```python
from build123d import *

# Parameters (mm, degrees)
F2_R = 12.7
F4_R = 2.54


# Not quite as in the source:
# - a fillet or chamfer that OpenCascade refuses, or shapes differently, is made with other operations: its cross-section is extruded or revolved along the edge and cut away or added


with BuildPart() as f1:
    # F0 (on Front) → F1 (revolve)
    with BuildSketch(Plane.XZ):
        Polygon((53.5, 27), (-30.1052267423, 27), (-40.7862067223, 8.5), (-48.5, 8.5), (-48.5, 10), (-53.5, 10), (-53.5, 6.5), (-39.6315061839, 6.5), (-28.9505262039, 25), (51.5, 25), (51.5, 0), (53.5, 0), align=None)
    revolve(axis=Axis((0, 0, 0), (1, 0, 0)))

    # F2
    f2_edges = [f1.edges().sort_by_distance(p)[0] for p in [
        (-30.105227, 0, -27),
        (-28.950526, 0, -25),
    ]]
    fillet(f2_edges, radius=F2_R)

    # F3: fillet of radius 5.08 on 2 edges, made by hand

    # F3_s1 → F3_t2 (revolve)
    with BuildSketch(Plane.XZ):
        with BuildLine():
            ThreePointArc((-43.7191460897, 8.5), (-41.1791460897, 9.1805909488), (-39.3197370385, 11.04))
            Line((-39.3197370385, 11.04), (-40.7862067223, 8.5))
            Line((-40.7862067223, 8.5), (-43.7191460897, 8.5))
        make_face()
    revolve(axis=Axis((-40.7862067223, 0, 0), (1, 0, 0)))

    # F3_s3 → F3_t4 (revolve)
    with BuildSketch(Plane.XZ):
        with BuildLine():
            ThreePointArc((-48.5, 10), (-46.8477578714, 8.8899680172), (-44.8958357418, 8.5))
            Line((-44.8958357418, 8.5), (-48.5, 8.5))
            Line((-48.5, 8.5), (-48.5, 10))
        make_face()
    revolve(axis=Axis((-48.5, 0, 0), (1, 0, 0)))

    # F4
    f4_edges = [f1.edges().sort_by_distance(p)[0] for p in [
        (-48.5, 0, -10),
        (-53.5, 0, -10),
    ]]
    fillet(f4_edges, radius=F4_R)

    # F5: fillet of radius 2.54 on 1 edges, made by hand

    # F5_s1 → F5_t2 (revolve, cut)
    with BuildSketch(Plane.XZ):
        with BuildLine():
            ThreePointArc((-53.5, 7.46), (-52.6154054362, 6.7525560116), (-51.5112315369, 6.5))
            Line((-51.5112315369, 6.5), (-53.5, 6.5))
            Line((-53.5, 6.5), (-53.5, 7.46))
        make_face()
    revolve(axis=Axis((-53.5, 0, 0), (1, 0, 0)), mode=Mode.SUBTRACT)


solid = f1.part
```
Check sheet for the modelled part. Datum: model origin and axes. Units: mm. A direction names the side the tool comes from. Coordinates: 2 decimals unless noted, no trailing zeros. Order: outer loops, then holes, each group sorted by start corner. A loop starts at its lowest first (then second) coordinate and runs counter-clockwise, first axis right, second up. Notation, with made-up numbers: M -20.5,5 L 38.5,5 A13 cw 38.5,30 Z; hole C 72,-8.75 d1. An arc over 180 degrees is marked long. Write each question's results on one line, items separated by ' | '. Start each with the question number.
1. Mould release check, pull along Z, two halves, no side actions. Record for faces 1 (the face through (-50.21, -3, 9.54)), 2 (the face through (15.453, -7.509, 23.846)), 3 (the face through (53.5, 0, 0)): +Z half, -Z half, draft (parallel to the pull), parting line (faces both ways), or undercut.
2. Cross-section at A-A on x = 18. Record the cut outline in (y, z).
3. Go/stop test with flat-tipped pins: P1, Ø1, axis at y = 10.5, z = 15.5, coming from the -X side; P2, Ø12, axis at x = -8.5, z = 13, coming from the +Y side; P3, Ø6, axis at x = 25, z = -3, coming from the -Y side; P4, Ø2, axis at y = -19, z = -21.5, coming from the -X side. Record where each tip stops, or that it passes through.
4. Access from +Z, -Z, +X, -X, +Y, -Y to the whole of each face (thin tool, end or side, straight path). Record for faces 4 (the face through (-44.316, -7.167, 4.57)), 5 (the face through (14.83, 26.36, -5.85)), 6 (the face through (-45.488, 3.955, -5.158)).
5. Material ranges on probe 1 along Z at (x, y) = (27, 0); probe 2 along Y at (x, z) = (-43.75, 0), recorded low to high.
Checks:
1) face 1: parting line | face 2: undercut | face 3: draft
2) outline: C 0,0 d54; hole C 0,0 d50
3) P1: stops at x = -35.17 | P2: stops at y = 26.08 | P3: stops at y = -27 | P4: passes through
4) face 4: none | face 5: +X, -X | face 6: -X
5) probe 1: z = -27 to -25, 25 to 27 | probe 2: y = -8.5 to -6.5, 6.5 to 8.5
